Verification items for the finished model (mm, model axes). A direction names the side the tool comes from. Coordinates: 2 decimals unless noted, no trailing zeros. Order: outer loops, then holes, each group sorted by start corner. A loop starts at its lowest first (then second) coordinate and runs counter-clockwise, first axis right, second up. Notation, with made-up numbers: (54, 54) -> (85, 54) arc R28 cw to (85, 93) -> close; hole circle Ø4 at (-8.5, 2). An arc over 180 degrees is marked (long way). Use CSV: the item, a comma, the result in double quotes. Start each with the question number.
1) Scan lines: line 1 along Y through (x, z) = (16, 21); line 2 along X through (y, z) = (-13, 21); line 3 along Z through (x, y) = (11, -23.5). Record each from-to range of solid material in increasing order.
2) Sectioned sample at A-A on z = 6. Record the boundary of the cut face in (x, y), then the cut area to 3 significant figures.
3) Sectioned sample at C-C on y = -12.5. Record the boundary of the cut face in (x, z), then the cut area to 3 significant figures.
4) Release check for a two-part mould opening along X. For faces 1 (the flat face through (24, -12, 4)), 2 (the flat face through (0, -12, 10)), 3 (the flat face through (-16, -20, 19)) record: released by +X, released by -X, zero draft, split by the parting line, or undercut.
5) Tool access check on faces 4 (the flat face through (-17, -12, 14)), 5 (the flat face through (-7.535, -12.325, 4.93)), 6 (the flat face through (16, -5, 19)), 7 (the cylindrical face through (-7.94, -18.58, 35.39)), 8 (the flat face through (0, -8.5, 38)). Record the directions out of +Z, -Z, +X, -X, +Y, -Y that give a thin tool (end or side, any length) a straight path to the whole face; none if there is none.
6) Sectioned sample at D-D on z = 19.5. Record the boundary of the cut face in (x, y) (3 decimals).
7) Go/stop test with flat-tipped pins: pin 1 (4 mm diameter, centred on y = -9.5, z = 23, fed in from +X); pin 2 (8 mm diameter, centred on x = 0, z = 39, fed in from -Y); pin 3 (3 mm diameter, centred on y = -19, z = 18, fed in from +X). Record where each tip stops, or that it passes through.
8) Sectioned sample at B-B on x = 0. Record the boundary of the cut face in (y, z).
from build123d import *

# Parameters (mm, degrees)
F1_DEPTH   = 25
F2_SIZE2   = 9
F2_SIZE    = 20
F2_2_SIZE2 = 9
F2_2_SIZE  = 20
F3_R       = 10
F4_DEPTH   = 15
F6_DEPTH   = 10
F7_W       = 15
F7_H       = 14
F8_DEPTH   = 11
F9_W       = 15
F9_H       = 14
F10_DEPTH  = 11


with BuildPart() as f1:
    # F0 (on Front) → F1 (new body)
    with BuildSketch(Plane.XZ):
        Polygon((24, 28), (-24, 28), (-24, 0), (-10, 0), (-5, 10), (5, 10), (10, 0), (24, 0), align=None)
    extrude(amount=F1_DEPTH)

    # F2
    f2_edges = [f1.edges().sort_by_distance(p)[0] for p in [
        (-24, -12.5, 28),
    ]]
    f2_side = f1.faces().sort_by_distance((-24, -12.5, 14))[0]
    chamfer(f2_edges, length=F2_SIZE, length2=F2_SIZE2, reference=f2_side)

    # F2#2
    f2_2_edges = [f1.edges().sort_by_distance(p)[0] for p in [
        (24, -12.5, 28),
    ]]
    f2_2_side = f1.faces().sort_by_distance((24, -12.5, 14))[0]
    chamfer(f2_2_edges, length=F2_2_SIZE, length2=F2_2_SIZE2, reference=f2_2_side)

    # F3 (on face) → F4 (join)
    with BuildSketch(Plane.XY.offset(28)):
        with Locations((0, -12.5)):
            Circle(F3_R)
    extrude(amount=F4_DEPTH)

    # F5 (on face) → F6 (cut)
    with BuildSketch(Plane.XY.offset(43)):
        with BuildLine():
            Line((9.1651513899, -8.5), (-9.1651513899, -8.5))
            ThreePointArc((-9.1651513899, -8.5), (-10, -12.5), (-9.1651513899, -16.5))
            Line((-9.1651513899, -16.5), (9.1651513899, -16.5))
            ThreePointArc((9.1651513899, -16.5), (9.7890631293, -14.5430964369), (10, -12.5))
            ThreePointArc((10, -12.5), (9.7890631293, -10.4569035631), (9.1651513899, -8.5))
        make_face()
    extrude(amount=-F6_DEPTH, mode=Mode.SUBTRACT)

    # F7 (on face) → F8 (cut)
    with BuildSketch(Plane.YZ.offset(24)):
        with Locations((-12.5, 21)):
            Rectangle(F7_W, F7_H)
    extrude(amount=-F8_DEPTH, mode=Mode.SUBTRACT)

    # F9 (on face) → F10 (cut)
    with BuildSketch(Plane(origin=(-24, 0, 0), x_dir=(0, -1, 0), z_dir=(-1, 0, 0))):
        with Locations((12.5, 21)):
            Rectangle(F9_W, F9_H)
    extrude(amount=-F10_DEPTH, mode=Mode.SUBTRACT)


solid = f1.part
Answers follow:
1,line 1,"y = -25 to -20, -5 to 0"
1,line 2,"x = -13 to 13"
1,line 3,"z = 0 to 28"
2,outline,"(-24, -25) -> (-7, -25) -> (-7, 0) -> (-24, 0) -> close; (7, -25) -> (24, -25) -> (24, 0) -> (7, 0) -> close"
2,area,"850 mm²"
3,outline,"(-24, 0) -> (-10, 0) -> (-5, 10) -> (5, 10) -> (10, 0) -> (24, 0) -> (24, 8) -> (21.3, 14) -> (13, 14) -> (13, 28) -> (10, 28) -> (10, 33) -> (-10, 33) -> (-10, 28) -> (-13, 28) -> (-13, 14) -> (-21.3, 14) -> (-24, 8) -> close"
3,area,"970 mm²"
4,face 1,"released by +X"
4,face 2,"undercut"
4,face 3,"zero draft"
5,face 4,"+Z, -X"
5,face 5,"-Z, +Y, -Y"
5,face 6,"+Z, +X"
5,face 7,"+Z"
5,face 8,"+Z, +X, -X"
6,outline,"(-18.825, -25) -> (18.825, -25) -> (18.825, -20) -> (13, -20) -> (13, -5) -> (18.825, -5) -> (18.825, 0) -> (-18.825, 0) -> (-18.825, -5) -> (-13, -5) -> (-13, -20) -> (-18.825, -20) -> close"
7,pin 1,"stops at x = 13"
7,pin 2,"stops at y = -22.5"
7,pin 3,"stops at x = 20"
8,outline,"(-25, 10) -> (0, 10) -> (0, 28) -> (-2.5, 28) -> (-2.5, 43) -> (-8.5, 43) -> (-8.5, 33) -> (-16.5, 33) -> (-16.5, 43) -> (-22.5, 43) -> (-22.5, 28) -> (-25, 28) -> close"
